```python
from build123d import *


with BuildPart() as part:
    # Sketch 1 → Revolve 1 (revolve)
    with BuildSketch(Plane.XY, mode=Mode.PRIVATE) as revolve_1_sk:
        with BuildLine():
            Line((1.1, 1.1), (1.1, 1.3465))
            Line((1.1, 1.3465), (1.2535, 1.5))
            Line((1.2535, 1.5), (19.1, 1.5))
            Line((19.1, 1.5), (19.1, 1.3465))
            Line((19.1, 1.3465), (20, 1.3465))
            Line((20, 1.3465), (20, 2.9))
            Line((20, 2.9), (20.6, 3.5))
            Line((20.6, 3.5), (22.4, 3.5))
            Line((22.4, 3.5), (23, 2.9))
            Line((23, 2.9), (23, 0))
            Line((23, 0), (0, 0))
            ThreePointArc((0, 0), (0.322182541, 0.777817459), (1.1, 1.1))
        make_face()
    revolve(revolve_1_sk.sketch.rotate(Axis((23, 0, 0), (-1, 0, 0)), 270), axis=Axis((23, 0, 0), (-1, 0, 0)))


solid = part.part
```
The model under review builds one solid part; all positions refer to its coordinate system, in mm. Give positions to 0.01 mm unless a question says otherwise; leave off trailing zeros. Write each loop counter-clockwise with the first axis right and the second up, starting at its lowest first coordinate (ties: lowest second). Pieces come first, ordered by that corner, then holes. Notation, with made-up numbers: (83, 6.5) - (121, 6.5) arc R25 ccw to (121, 33.5) - close; hole circle Ø3 at (71, 15). An arc over 180 degrees is marked (long way). Answer in a Markdown table with one row per item. Add a question column.
1. We need section A-A on z = 0. Write out the cut boundary in (x, y), then the cut area to 3 significant figures.
2. We need section C-C on x = 15. Write out the cut boundary in (y, z), then the cut area to 3 significant figures.
3. Wall thickness on line 1 along X through (y, z) = (-2.25, 0.25); line 2 along Y through (x, z) = (18.5, 0.25); line 3 along Y through (x, z) = (21, -2): over which ranges is each line inside the solid? List them lowest first. Write a range as [from, to].
4. Insertion check: P1, Ø4, axis at y = -1, z = -2.5, coming from the -X side; P2, Ø1.5, axis at x = 8.5, z = 0.5, coming from the -Y side; P3, Ø0.8, axis at y = 0, z = 0.5, coming from the -X side. Each pin has a flat end and moves straight along its axis. Give the tip position at first contact, or say it passes through.
5. Draft analysis for pull direction X (two halves, no side actions). For faces 1 (the flat face through (23, 0, 0)), 2 (the cylindrical face through (10.3, 0.45, 1.43)), 3 (the cylindrical face through (19.556, 0.404, 1.284)), state which applies: +X half, -X half, draft (parallel to the pull), parting line (faces both ways), or undercut.
Ans:
| question | item | result |
|---|---|---|
| 1 | outline | (1.1, -1.35) - (1.25, -1.5) - (19.1, -1.5) - (19.1, -1.35) - (20, -1.35) - (20, -2.9) - (20.6, -3.5) - (22.4, -3.5) - (23, -2.9) - (23, 2.9) - (22.4, 3.5) - (20.6, 3.5) - (20, 2.9) - (20, 1.35) - (19.1, 1.35) - (19.1, 1.5) - (1.25, 1.5) - (1.1, 1.35) - (1.1, 1.1) arc R1.1 ccw to (1.1, -1.1) - close |
| 1 | area | 78.6 mm^2 |
| 2 | outline | circle Ø3 at (0, 0) |
| 2 | area | 7.07 mm^2 |
| 3 | line 1 | x = [20, 23] |
| 3 | line 2 | y = [-1.48, 1.48] |
| 3 | line 3 | y = [-2.87, 2.87] |
| 4 | P1 | stops at x = 0.25 |
| 4 | P2 | stops at y = -1.5 |
| 4 | P3 | stops at x = 0 |
| 5 | face 1 | +X half |
| 5 | face 2 | draft |
| 5 | face 3 | undercut |
